The model under review builds one solid part; all positions refer to its coordinate system, in mm. A direction names the side the tool comes from. Round coordinates to 2 decimals unless told otherwise and drop trailing zeros. Loops run counter-clockwise (first coordinate to the right, second up) from the corner with the lowest first, then second, coordinate; pieces in that order, holes last. Notation, with made-up numbers: M 18,65.25 L 77,65.25 A22 cw 77,94.25 Z; hole C 63.5,-20.75 d11. An arc over 180 degrees is marked long. Return JSON: item names as keys, results as strings. Group by question number.
Q1. Draft analysis for pull direction X (two halves, no side actions). For faces 3 (the face through (-32.034, -47.156, 3.479)), 4 (the face through (-19, -23, 5)), 5 (the face through (-28.14, -44.37, 4.51)), state which applies: pulls with the +X half, pulls with the -X half, needs draft (parallel to the pull), parting line crosses it, or undercut.
Q2. Clearance check with flat-ended pins moving along their axes: pin 1 Ø0.5 at (y, z) = (-18.5, 4.5) entering from +X; pin 2 Ø2 at (y, z) = (-43, 4) entering from -X; pin 3 Ø2 at (x, y) = (-25.5, -33) entering from +Z. State where each tip first meets the part, or that it passes through.
Q3. To check wall thickness, follow line 1 along Z through (x, y) = (-7.5, -32); line 2 along Z through (x, y) = (-36, -38); line 3 along Y through (x, z) = (-24.5, 4.7). State the ranges of each line that lie inside material, in increasing order.
Q4. For faces 1 (the face through (-23, -30, 5)), 2 (the face through (-22.027, -19.14, 4.507)), list the 3-axis set-ups (+Z, -Z, +X, -X, +Y, -Y) from which the entire face can be reached by the end or side of a thin tool; tool diameter is ignored.
Q5. Consider section B-B (x = -9). State the section outline as (y, z) points, and give its area (3 significant figures).
Q6. Consider section A-A (y = -36). State the section outline as (x, z) points, and give its area (3 significant figures).
Q7. Consider section D-D (y = -19). State the section outline as (x, z) points, and give its area (3 significant figures).
Q8. Consider section C-C (z = 3.3). State the section outline as (x, y) points.
from build123d import *

# Parameters (mm, degrees)
SKETCH027_R     = 22.5
PAD008_DEPTH    = 2
SKETCH028_R     = 19.75
PAD009_DEPTH    = 3
POCKET014_DEPTH = 1
SKETCH030_R     = 2.75
PAD010_DEPTH    = 1


with BuildPart() as part:
    # Sketch027 → Pad008 (new body)
    with BuildSketch(Plane.XY):
        with Locations((-27.752922, -27.875624)):
            Circle(SKETCH027_R)
    extrude(amount=PAD008_DEPTH)

    # Sketch028 (on Face3 of Pad008) → Pad009 (join)
    with BuildSketch(Plane.XY.offset(2)):
        with Locations((-27.752922, -27.875624)):
            Circle(SKETCH028_R)
    extrude(amount=PAD009_DEPTH)

    # Sketch029 (on Face5 of Pad009) → Pocket014 (cut)
    with BuildSketch(Plane.XY.offset(5)):
        with BuildLine():
            ThreePointArc((-34.368184, -24.587091), (-27.755113, -44.375624), (-21.134159, -24.589727))
            Line((-16.118527, -17.931863), (-21.134159, -24.589727))
            ThreePointArc((-16.118527, -17.931863), (-16.443912, -15.185115), (-19.202253, -15.39019))
            Line((-24.774256, -22.786594), (-19.202253, -15.39019))
            ThreePointArc((-24.774256, -22.786594), (-25.260988, -22.661602), (-25.752922, -22.55897))
            Line((-25.752922, -12.875624), (-25.752922, -22.55897))
            ThreePointArc((-25.752922, -12.875624), (-27.752922, -10.875624), (-29.752922, -12.875624))
            Line((-29.752922, -12.875624), (-29.752922, -22.55897))
            ThreePointArc((-29.752922, -22.55897), (-30.242757, -22.661114), (-30.727441, -22.785429))
            Line((-36.191966, -15.525677), (-30.727441, -22.785429))
            ThreePointArc((-36.191966, -15.525677), (-39.061624, -15.184862), (-39.276171, -18.066713))
            Line((-39.276171, -18.066713), (-34.368184, -24.587091))
        make_face()
    extrude(amount=-POCKET014_DEPTH, mode=Mode.SUBTRACT)

    # Sketch030 (on Face18 of Pocket014) → Pad010 (join)
    with BuildSketch(Plane.XY.offset(4)):
        with Locations((-22.574881, -29.54578)):
            Circle(SKETCH030_R)
    extrude(amount=PAD010_DEPTH)


solid = part.part
Values:
{
 "1": {"face 3": "parting line crosses it", "face 4": "needs draft", "face 5": "undercut"},
 "2": {"pin 1": "stops at x = -10.24", "pin 2": "stops at x = -41.56", "pin 3": "stops at z = 4"},
 "3": {"line 1": "z = 0 to 2", "line 2": "z = 0 to 4", "line 3": "y = -47.36 to -43.88, -31.51 to -27.58, -22.42 to -8.4"},
 "4": {"face 1": "+Z, +X, -X, +Y, -Y", "face 2": "+Z"},
 "5": {"outline": "M -40.31,0 L -15.44,0 L -15.44,2 L -21.68,2 L -21.68,5 L -34.07,5 L -34.07,2 L -40.31,2 Z", "area": "86.9 mm2"},
 "6": {"outline": "M -48.73,0 L -6.77,0 L -6.77,2 L -9.75,2 L -9.75,5 L -17.07,5 L -17.07,4 L -38.44,4 L -38.44,5 L -45.75,5 L -45.75,2 L -48.73,2 Z", "area": "171 mm2"},
 "7": {"outline": "M -48.43,0 L -7.08,0 L -7.08,2 L -10.11,2 L -10.11,5 L -16.92,5 L -16.92,4 L -21.92,4 L -21.92,5 L -25.75,5 L -25.75,4 L -29.75,4 L -29.75,5 L -33.58,5 L -33.58,4 L -38.57,4 L -38.57,5 L -45.4,5 L -45.4,2 L -48.43,2 Z", "area": "175 mm2"},
 "8": {"outline": "C -27.75,-27.88 d39.5"}
}
